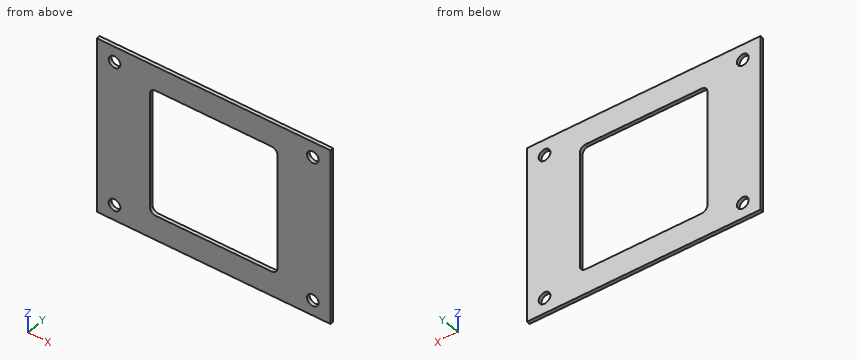
from build123d import *

# Parameters (mm, degrees)
SKETCH1_W           = 66
SKETCH1_H           = 50
SKETCH1_R           = 1.65
SKETCH1_W_2         = 36
SKETCH1_H_2         = 36
BOSS_EXTRUDE1_DEPTH = 1
FILLET1_R           = 1.6


with BuildPart() as part:
    # Sketch1 → Boss-Extrude1 (new body)
    with BuildSketch(Plane(origin=(0, 0, 0), x_dir=(1, 0, 0), z_dir=(0, 1, 0))):
        Rectangle(SKETCH1_W, SKETCH1_H)
        with Locations((-28, 20.6)):
            Circle(SKETCH1_R, mode=Mode.SUBTRACT)
        with Locations((-28, -20.6)):
            Circle(SKETCH1_R, mode=Mode.SUBTRACT)
        with Locations((28, 20.6)):
            Circle(SKETCH1_R, mode=Mode.SUBTRACT)
        with Locations((28, -20.6)):
            Circle(SKETCH1_R, mode=Mode.SUBTRACT)
        Rectangle(SKETCH1_W_2, SKETCH1_H_2, mode=Mode.SUBTRACT)
    extrude(amount=BOSS_EXTRUDE1_DEPTH)

    # Fillet1
    fillet1_edges = [part.edges().sort_by_distance(p)[0] for p in [
        (18, 0.5, 18),
        (18, 0.5, -18),
        (-18, 0.5, -18),
        (-18, 0.5, 18),
    ]]
    fillet(fillet1_edges, radius=FILLET1_R)


solid = part.part
The listing builds one solid part. Answer for the finished solid, in the listing's coordinates (mm). Coordinates: 2 decimals unless noted, no trailing zeros. Loops run counter-clockwise (first coordinate to the right, second up) from the corner with the lowest first, then second, coordinate; pieces in that order, holes last. Notation, with made-up numbers: (60.25, 67) -> (95.25, 67) arc R31 ccw to (95.25, 96) -> close; hole circle Ø4 at (-8.75, -5). An arc over 180 degrees is marked (long way). Answer in a Markdown table with one row per item. Add a question column.
1. Consider line 1 (Z direction, x = -28, y = 0.85); line 2 (X direction, y = 0.6, z = 20.6); line 3 (Z direction, x = 13.5, y = 0.6). Determine where each line is inside the solid, lowest interval first. Write a range as [from, to].
2. The part is cut by section D-D, the plane z = 20.6. Write down the section's boundary in (x, y), then the cut area to 3 significant figures.
3. The part is cut by section B-B, the plane z = -12. Write down the section's boundary in (x, y), then the cut area to 3 significant figures.
4. The part is cut by section A-A, the plane x = -13.5. Write down the section's boundary in (y, z).
5. A flat-ended cylindrical pin translates along its axis: P1, Ø2, axis at x = -28, z = -20.6, coming from the +Y side. Find the tip coordinate at first contact, or state that the pin passes through.
6. The part is cut by section C-C, the plane x = -28. Write down the section's boundary in (y, z).
Answer below:
| question | item | result |
|---|---|---|
| 1 | line 1 | [-25, -22.25], [-18.95, 18.95], [22.25, 25] |
| 1 | line 2 | [-33, -29.65], [-26.35, 26.35], [29.65, 33] |
| 1 | line 3 | [-25, -18], [18, 25] |
| 2 | outline | (-33, 0) -> (-29.65, 0) -> (-29.65, 1) -> (-33, 1) -> close; (-26.35, 0) -> (26.35, 0) -> (26.35, 1) -> (-26.35, 1) -> close; (29.65, 0) -> (33, 0) -> (33, 1) -> (29.65, 1) -> close |
| 2 | area | 59.4 mm2 |
| 3 | outline | (-33, 0) -> (-18, 0) -> (-18, 1) -> (-33, 1) -> close; (18, 0) -> (33, 0) -> (33, 1) -> (18, 1) -> close |
| 3 | area | 30.0 mm2 |
| 4 | outline | (0, -25) -> (1, -25) -> (1, -18) -> (0, -18) -> close; (0, 18) -> (1, 18) -> (1, 25) -> (0, 25) -> close |
| 5 | P1 | through |
| 6 | outline | (0, -25) -> (1, -25) -> (1, -22.25) -> (0, -22.25) -> close; (0, -18.95) -> (1, -18.95) -> (1, 18.95) -> (0, 18.95) -> close; (0, 22.25) -> (1, 22.25) -> (1, 25) -> (0, 25) -> close |
